Read the model definition and answer for the solid it produces. Units are mm, in the model's axes. Give positions to 0.01 mm unless a question says otherwise; leave off trailing zeros. Loops run counter-clockwise (first coordinate to the right, second up) from the corner with the lowest first, then second, coordinate; pieces in that order, holes last. Notation, with made-up numbers: (-25.75, 56.25) - (26.25, 56.25) arc R17 ccw to (26.25, 64.25) - close; hole circle Ø1 at (7, 61.5). An arc over 180 degrees is marked (long way). Write item = value, one per line.
Autodesk Inventor part; units mm, degrees
ref_plane "YZ Plane" through (0, 0, 0) normal (1, 0, 0) x (0, 1, 0)
ref_plane "XZ Plane" through (0, 0, 0) normal (0, 1, 0) x (-1, 0, 0)
ref_plane "XY Plane" through (0, 0, 0) normal (0, 0, 1) x (1, 0, 0)
sketch "Esquisse1" plane through (0, 0, 0) normal (1, 0, 0) x (0, 1, 0)
  line L0 (0, -56) -> (0, 56)
  line L1 (-49.4, 0) -> (30.4, 0)
  line L2 (-47.5, 32) -> (-47.5, 0)
  line L3 (23.32, 200.2) -> (-20.32, 200.2)
  line L4 (-50.5, 0) -> (-50.5, 32)
  line L5 (-47.5, 0) -> (-50.5, 0)
  line L6 (-50.5, 0) -> (-47.5, 0)
  line L7 (-47.5, 32) -> (-50.5, 32) construction
  line L8 (-47.5, -30) -> (-47.5, 30)
  line L9 (-17.32, -203.2) -> (-17.32, 203.2) construction
  line L10 (-20.32, -203.2) -> (-20.32, 203.2) construction
  line L11 (18.32, 203.2) -> (18.32, -203.2) construction
  line L12 (17.32, -203.2) -> (17.32, 203.2) construction
  line L13 (20.32, -203.2) -> (20.32, 203.2) construction
  line L14 (20.32, 215.2) -> (23.32, 215.2)
  line L15 (23.32, 215.2) -> (23.32, 200.2)
  line L16 (-23.32, 200.2) -> (-23.32, 215.2)
  line L17 (-23.32, 215.2) -> (-20.32, 215.2)
  line L18 (-20.32, 215.2) -> (-20.32, 203.2)
  line L19 (-20.32, 203.2) -> (20.32, 203.2)
  line L20 (20.32, 203.2) -> (20.32, 215.2)
  line L21 (-20.32, 200.2) -> (-23.32, 200.2) construction
  line L22 (20.32, 203.2) -> (20.32, 200.2) construction
  line L23 (-20.32, 200.2) -> (-20.32, 180.2) construction
  line L24 (-20.32, 180.2) -> (-33.0773, 176.0923) construction
  line L25 (-33.0773, 176.0923) -> (-50, 129.3731) construction
  line L26 (-50, 129.3731) -> (-47.5, 42) construction
  line L27 (-47.5, 42) -> (-47.5, 32) construction
  spline S0 degree 4 poles (-20.32, 200.2) (-20.32, 180.2) (-33.0773, 176.0923) (-50, 129.3731) (-47.5, 42) (-47.5, 32) knots 1 1 1 1 1 2 3 3 3 3 3
  spline S1 degree 5 poles (-23.32, 200.2) (-23.3199, 198.3844) (-23.3716, 196.5688) (-23.4859, 194.7552) (-23.8349, 191.6186) (-24.5084, 188.5383) (-24.8603, 187.248) (-25.6789, 184.7885) (-26.7147, 182.4126) (-27.2583, 181.281) (-28.4715, 178.8909) (-29.747, 176.5332) (-30.4258, 175.2799) (-31.9037, 172.5044) (-33.3133, 169.6936) (-34.0545, 168.1423) (-35.6303, 164.6693) (-37.0531, 161.1305) (-37.7885, 159.1688) (-39.3183, 154.8027) (-40.6538, 150.3728) (-41.332, 147.9334) (-42.7081, 142.5835) (-43.8774, 137.1842) (-44.457, 134.2482) (-45.5952, 127.9452) (-46.5359, 121.6095) (-46.9881, 118.227) (-47.8405, 111.1566) (-48.5208, 104.0676) (-48.8338, 100.3717) (-49.3914, 92.8899) (-49.8093, 85.3989) (-49.9882, 81.6095) (-50.2781, 74.2453) (-50.4635, 66.8779) (-50.5309, 63.3022) (-50.6147, 56.7606) (-50.6326, 50.2184) (-50.6275, 47.2525) (-50.6011, 42.4224) (-50.5494, 37.5925) (-50.531, 35.7284) (-50.5018, 33.8642) (-50.5, 32) knots 0 0 0 0 0 0 0.052645 0.052645 0.052645 0.091341 0.091341 0.091341 0.127725 0.127725 0.127725 0.169058 0.169058 0.169058 0.218895 0.218895 0.218895 0.27962 0.27962 0.27962 0.353015 0.353015 0.353015 0.439772 0.439772 0.439772 0.538713 0.538713 0.538713 0.646254 0.646254 0.646254 0.75625 0.75625 0.75625 0.859944 0.859944 0.859944 0.945945 0.945945 0.945945 1 1 1 1 1 1
  point P0 (0, 0)
  point P1 (-20.32, 200.2)
  dimension "d9" = 3
  dimension "d16" = 203.2
  dimension "d17" = 12
  dimension "d19" = 32
  dimension "d21" = 20
  dimension "d22" = 10
revolve "Révolution1" add sketch "Esquisse1" angle 360 about axis through (0, -49.4, 0) along (0, 1, 0)
sketch "Esquisse2" plane through (0, 0, 0) normal (0, 1, 0) x (-1, 0, 0)
  circle A0 centre (11, 19.0526) radius 2.5
  circle A1 centre (-11, 19.0526) radius 2.5
  circle A2 centre (-22, 0) radius 2.5
  circle A3 centre (-11, -19.0526) radius 2.5
  circle A4 centre (11, -19.0526) radius 2.5
  circle A5 centre (22, 0) radius 2.5
  circle A6 centre (-11, -19.0526) radius 2.5
  circle A7 centre (11, -19.0526) radius 2.5
  circle A8 centre (22, 0) radius 2.5
  circle A9 centre (11, 19.0526) radius 2.5
  circle A10 centre (-11, 19.0526) radius 2.5
  circle A11 centre (-22, 0) radius 2.5
  circle A12 centre (0, 0) radius 30
  circle A13 centre (0, 0) radius 13
  point P0 (0, 0)
extrude "Extrusion1" cut sketch "Esquisse2" against normal through all contours A0 | A1 | A2 | A3 | A4 | A5
fillet "Congé1" [suppressed]
fillet "Congé3" radius 7.25 1 edges at (0, -20.32, -200.2)
equation "\"d_profile_section\" = 40"
equation "\"d_prfc_thickness\" = 3"
equation "\"d_arm_in_diameter\" = 27"
equation "\"d_arm_out_diameter\" = 30"
equation "\"d_arm_length\" = 250"
equation "\"d_suspension_height\" = 140"
equation "\"d_aluminum_thickness\" = 3.175"
equation "\"d_suspension_box_width\" = 40"
equation "\"d_wheelbase\" = 1600"
equation "\"a_tilt\" = 10deg"
equation "\"d_rear_profile_height\" = 101.6"
equation "\"d_rear_profile_width\" = 50.8"
equation "\"d_central_profile_width\" = 50.8"
equation "\"d_central_profile_height\" = 101.6"
equation "\"d_handle_bar_tube_diameter\" = 35"
equation "\"a_direction_column\" = 35deg"
equation "\"prfc_tube_id\" = 33"
equation "\"prfc_tube_od\" = 35"
equation "\"front_suspension_height\" = 140.92977"
equation "\"front_suspension_width\" = 150"
equation "\"caster_angle\" = 24deg"
equation "\"a_caster_angle\" = 25deg"
equation "\"d_handlebar_pivot_offset\" = 65"
equation "\"d_handlebar_arm_length\" = 80"
equation "\"a_handlebar_angle\" = 60deg"
equation "\"d_left_to_right_front_pivots\" = 28"
equation "\"d_front_arm_id\" = 29.2608"
equation "\"d_front_arm_od\" = 31.75"
equation "\"d_aluminum_bar_thickness\" = 12.7"
equation "\"d_handle_bar_id\" = 30"
equation "\"d_handle_bar_od\" = 38.1"
equation "\"d_steering_arm_length\" = 70"
equation "\"d_steering_height_from_hub_center\" = 28"
equation "\"d_steering_height_from_hub_carrier_center\" = 18"
equation "\"d_central_beam_inclination\" = 12"
equation "\"a_central_beam_inclination\" = 12deg"
equation "\"d_central_beam_screws_diameter\" = 8"
equation "\"d_rear_profile_wall_thickness\" = 4.7625"
equation "\"d_rear_profile_wall_thickness_1\" = 4.7625"
equation "\"d_central_pivot_screw_diameter\" = 15.875"
properties part number "wheel_rim" material "CFRP"
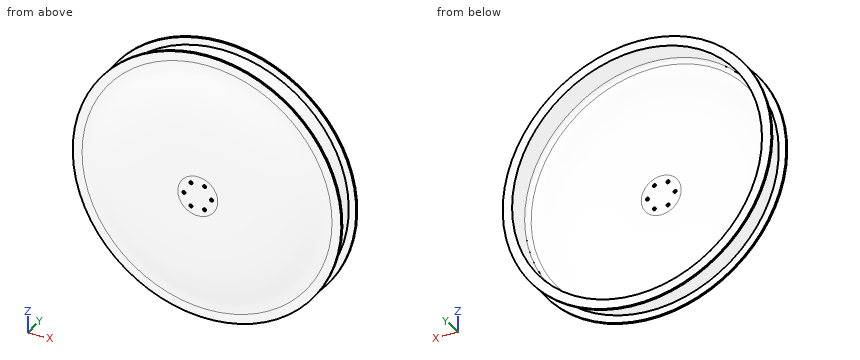
1) A cutting plane is placed at A-A on y = -6.5. Determine the outline of the cut face in (x, z), then the cut area to 3 significant figures.
Output:
outline = circle Ø406.4 at (0, 0); hole circle Ø400.4 at (0, 0)
area = 3,800 mm²
2) Find the intervals of material crossed by probe 1 along X at (y, z) = (15.5, 0); probe 2 along Y at (x, z) = (-164, 133); probe 3 along Z at (x, y) = (-6, -12), in increasing order.
Output:
probe_1 = -203.2 to -200.2, 200.2 to 203.2
probe_2 = -23.32 to -20.32, 20.32 to 23.32
probe_3 = -203.11 to -200.11, 200.11 to 203.11
3) Each of these flat-tipped pins is pushed along its axis until it touches: P1, Ø1.5, axis at x = -61.5, y = 12, coming from the +Z side; P2, Ø8, axis at x = -11, z = -19.05, coming from the +Y side; P3, Ø12, axis at x = 69.5, y = -7, coming from the +Z side. Where does it stop, or does it pass through?
Output:
P1 = 193.91
P2 = -47.5
P3 = 193.02
